Autodesk Inventor part; units mm, degrees
ref_plane "YZ Plane" through (0, 0, 0) normal (1, 0, 0) x (0, 1, 0)
ref_plane "XZ Plane" through (0, 0, 0) normal (0, 1, 0) x (-1, 0, 0)
ref_plane "XY Plane" through (0, 0, 0) normal (0, 0, 1) x (1, 0, 0)
sketch "Sketch1" plane through (0, 0, 0) normal (0, 0, 1) x (1, 0, 0)
  line L0 (0, 0) -> (1.778, 0)
  line L1 (1.778, 0) -> (1.778, 5.08)
  line L2 (1.778, 5.08) -> (0, 5.08)
  line L3 (0, 5.08) -> (0, 0)
  line L4 (1.778, 0) -> (11.049, 0)
  line L5 (11.049, 0) -> (11.049, 3.683)
  line L6 (11.049, 3.683) -> (1.778, 3.683)
  line L7 (1.778, 3.683) -> (1.778, 0)
  line L8 (8.509, 3.683) -> (6.985, 3.81)
  line L9 (6.985, 3.81) -> (6.985, 3.683)
  line L10 (6.985, 3.683) -> (5.461, 3.81)
  line L11 (5.461, 3.81) -> (5.461, 3.683)
  line L12 (5.461, 3.683) -> (3.937, 3.81)
  line L13 (3.937, 3.81) -> (3.937, 3.683)
  line L14 (0, 0) -> (0, 3.1252)
  line L15 (0, 3.81) -> (0.889, 3.81) construction
  line L16 (0, 3.81) -> (0, 0)
  arc A0 (0, 3.81) -> (-9.906, 3.556) centre (0, -189.484) ccw
  line L17 (-9.906, 3.556) -> (-9.906, 3.81)
  line L18 (-9.906, 3.81) -> (-11.176, 3.81)
  line L19 (-11.176, 3.81) -> (-11.176, 0)
  line L20 (-11.176, 0) -> (0, 0)
  dimension "d0" = 1.778
  dimension "d1" = 10.16
  dimension "d2" = 9.271
  dimension "d3" = 7.366
  dimension "d4" = 7.62
  dimension "d5" = 2.54
  dimension "d6" = 1.524
  dimension "d7" = 7.62
  dimension "d8" = 7.62
  dimension "d9" = 11.176
  dimension "d10" = 7.112
  dimension "d11" = 1.27
revolve "Revolution1" add sketch "Sketch1" angle 360 about axis through (-11.176, 0, 0) along (1, 0, 0)
sketch "Sketch2" plane through (0, 0, 0) normal (0, 0, 1) x (1, 0, 0)
  line L0 (-11.176, 0.508) -> (-6.096, 0.508)
  line L1 (-6.096, 0.508) -> (-6.096, -0.508)
  line L2 (-6.096, -0.508) -> (-11.176, -0.508)
  line L3 (-11.176, -0.508) -> (-11.176, 0.508)
  line L4 (-11.176, -3.81) -> (-11.176, 3.81) construction
  point P0 (0, 0)
  point P1 (-11.176, 0)
  dimension "d13" = 1.016
  dimension "d14" = 5.08
extrude "Extrusion1" cut sketch "Sketch2" along normal through all both and the other way through all
hole "Hole1" at (-11.176, 0, 0) direction (1, 0, 0) diameter 4.7625 depth 11.1125 counterbore diameter 6.35 counterbore depth 6.35
hole "Hole2" at (11.049, 0, 0) direction (-1, 0, 0) diameter 4.7625 depth 9.525 counterbore diameter 6.35 counterbore depth 1.27
equation "\"d8\" = d7"
properties part number "T9 Axle"
Can you work these out from the model? Positions are in its coordinate system, mm. A direction names the side the tool comes from. Coordinates: 2 decimals unless noted, no trailing zeros. Write each loop counter-clockwise with the first axis right and the second up, starting at its lowest first coordinate (ties: lowest second). Pieces come first, ordered by that corner, then holes. Notation, with made-up numbers: (10.5, 43.25) - (60.5, 43.25) arc R28 ccw to (60.5, 69.25) - close; hole circle Ø4 at (10.5, 61). An arc over 180 degrees is marked (long way). Return JSON: item names as keys, results as strings.
Q1. Thinking about a two-plate mould opening in X: for faces 4 (the cylindrical face through (10.41, 3.1, 0.69)), 5 (the flat face through (1.524, 0, 0)), 6 (the flat face through (-0.064, 0, 0)), which applies, +X half, -X half, draft (parallel to the pull), parting line (faces both ways), or undercut?
Computed values:
{"face 4": "draft", "face 5": "+X half", "face 6": "-X half"}
Q2. If we section it at A-A (x = 4.5): Please give me the cut outline in (y, z).
Computed values:
{"outline": "circle Ø7.53 at (0, 0); hole circle Ø4.76 at (0, 0)"}
Q3. If we section it at B-B (z = 4.75): Please give me the cut outline in (x, y), then the cut area to 3 significant figures.
Computed values:
{"outline": "(0, -1.8) - (1.78, -1.8) - (1.78, 1.8) - (0, 1.8) - close", "area": "6.40 mm2"}
Q4. Please list where these lines run through material, in increasing order: L1, parallel to Z at x = -3.55, y = 0; L2, parallel to X at y = 4, z = 2.75; L3, parallel to Y at x = 4, z = 0. Write a range as from..to.
Computed values:
{"L1": "z = -3.78..-2.38, 2.38..3.78", "L2": "x = 0..1.78", "L3": "y = -3.8..-2.38, 2.38..3.8"}
Q5. I'm going to push flat-ended pins straight in: pin 1 Ø1.5 at (x, z) = (-5, 1) entering from -Y; pin 2 Ø0.5 at (x, z) = (-9.5, -3.5) entering from +Y; pin 3 Ø0.5 at (x, z) = (-7.5, 3.5) entering from -Y. Where does each tip first touch, or does it pass through?
Computed values:
{"pin 1": "stops at y = -3.74", "pin 2": "stops at y = 1.49", "pin 3": "stops at y = -1.69"}
Q6. On a 3-axis mill with a long thin cutter (end or side, diameter ignored), from which of +Z, -Z, +X, -X, +Y, -Y can I reach the whole of each face in a straight line? I mean faces 1 (the cylindrical face through (-2.41, 1.45, -1.89)), 2 (the cylindrical face through (-10.55, -3.81, -0.08)), 3 (the cylindrical face through (9.761, 1.699, 3.267)). Say none if no direction works.
Computed values:
{"face 1": "-X", "face 2": "-X, -Y", "face 3": "+X"}
